For this review, take the finished solid that the model builds, in its own axes (mm). A direction names the side the tool comes from. Coordinates: 2 decimals unless noted, no trailing zeros. Loops run counter-clockwise (first coordinate to the right, second up) from the corner with the lowest first, then second, coordinate; pieces in that order, holes last.
1. To check wall thickness, follow probe 1 along X at (y, z) = (0.9, -50); probe 2 along X at (y, z) = (2.15, -27.5); probe 3 along X at (y, z) = (0.8, -27.5). State the ranges of each line that lie inside material, in increasing order.
2. Clearance check with flat-ended pins moving along their axes: P1, Ø1.6, axis at x = 35, z = -4, coming from the +Y side; P2, Ø1, axis at y = 0.5, z = -25, coming from the +X side; P3, Ø10, axis at x = 48.5, z = 5.5, coming from the +Y side; P4, Ø0.8, axis at y = 0.5, z = -22, coming from the -X side. State where each tip first meets the part, or that it passes through.
3. Take a section at B-B, the plane x = 9. State the section outline as (y, z) points, then the cut area to 3 significant figures.
4. Machinability: for faces 5 (the face through (70, 1, -31.9)), 6 (the face through (72, 0.125, -30)), 7 (the face through (-1, 1.2, -28)), which of the approach directions +Z, -Z, +X, -X, +Y, -Y give a long, thin tool a straight path to every point of the face, cutting with its end or side? Answer none if there is none.
5. Take a section at C-C, the plane y = 2.3. State the section outline as (x, z) points, then the cut area to 3 significant figures.
6. Take a section at A-A, the plane z = -27.5. State the section outline as (x, y) points (3 decimals).
7. Take a section at D-D, the plane x = 32.73. State the section outline as (y, z) points (3 decimals), then the cut area to 3 significant figures.
8. Mouldability with a two-part tool opening along Z and no side actions: class faces 1 (the face through (34, 1.5, -50)), 2 (the face through (76.15, 1.46, -27.4)), 3 (the face through (28.33, 1, 6)), 4 (the face through (70, 1, -23.1)) as pulls with the +Z half, pulls with the -Z half, needs draft (parallel to the pull), parting line crosses it, or undercut.
```python
from build123d import *

# Parameters (mm, degrees)
SKETCH1_W           = 68.5
SKETCH1_H           = 55
BOSS_EXTRUDE1_DEPTH = 1.5
SKETCH2_W           = 68.5
SKETCH2_H           = 55
SKETCH2_W_2         = 64.5
SKETCH2_H_2         = 51
BOSS_EXTRUDE2_DEPTH = 1.25
SKETCH3_R           = 1.25
SKETCH3_W           = 64.5
SKETCH3_H           = 40
CUT_EXTRUDE1_DEPTH  = 1.5
SKETCH4_W           = 23
SKETCH4_H           = 1.2
CUT_EXTRUDE2_DEPTH  = 3
SKETCH5_R           = 1.9
BOSS_EXTRUDE3_DEPTH = 2.625
SKETCH5_5_R         = 1.9
BOSS_EXTRUDE4_DEPTH = 1.55
BOSS_EXTRUDE5_DEPTH = 1.2


with BuildPart() as part:
    # Sketch1 → Boss-Extrude1 (new body)
    with BuildSketch(Plane(origin=(0, 0, 0), x_dir=(1, 0, 0), z_dir=(0, 1, 0))):
        with Locations((34.25, 27.5)):
            Rectangle(SKETCH1_W, SKETCH1_H)
    extrude(amount=BOSS_EXTRUDE1_DEPTH)

    # Sketch2 → Boss-Extrude2 (add)
    with BuildSketch(Plane(origin=(0, 1.5, 0), x_dir=(1, 0, 0), z_dir=(0, 1, 0))):
        with Locations((34.25, 27.5)):
            Rectangle(SKETCH2_W, SKETCH2_H)
        with Locations((34.25, 27.5)):
            Rectangle(SKETCH2_W_2, SKETCH2_H_2, mode=Mode.SUBTRACT)
    extrude(amount=BOSS_EXTRUDE2_DEPTH)

    # Sketch3 → Cut-Extrude1 (cut)
    with BuildSketch(Plane(origin=(0, 1.5, 0), x_dir=(1, 0, 0), z_dir=(0, 1, 0))):
        with Locations(Location((5, 50, 0), (0, 0, 270))):
            Circle(SKETCH3_R)
        with Locations(Location((63.5, 50, 0), (0, 0, 270))):
            Circle(SKETCH3_R)
        with Locations(Location((63.5, 5, 0), (0, 0, 270))):
            Circle(SKETCH3_R)
        with Locations(Location((5, 5, 0), (0, 0, 270))):
            Circle(SKETCH3_R)
        with Locations((34.25, 27.5)):
            Rectangle(SKETCH3_W, SKETCH3_H)
    extrude(amount=-CUT_EXTRUDE1_DEPTH, mode=Mode.SUBTRACT)

    # Sketch4 → Cut-Extrude2 (cut)
    with BuildSketch(Plane.ZY):
        with Locations((-27.5, 0.6)):
            Rectangle(SKETCH4_W, SKETCH4_H)
    extrude(amount=-CUT_EXTRUDE2_DEPTH, mode=Mode.SUBTRACT)

    # Sketch5 → Boss-Extrude3 (add)
    # profile 1 of 3: a face of its own
    with BuildSketch(Plane(origin=(0, 2.75, 0), x_dir=(1, 0, 0), z_dir=(0, 1, 0))):
        with BuildLine():
            Line((37.13, -11.52), (37.13, 0))
            Line((37.13, 0), (28.33, 0))
            Line((28.33, 0), (28.33, -11.52))
            ThreePointArc((28.33, -11.52), (32.73, -15.92), (37.13, -11.52))
        make_face()
        with Locations(Location((32.73, -11.52, 0), (0, 0, 270))):
            Circle(SKETCH5_R, mode=Mode.SUBTRACT)
    # profile 2 of 3: a face of its own
    with BuildSketch(Plane(origin=(0, 2.75, 0), x_dir=(1, 0, 0), z_dir=(0, 1, 0))):
        with BuildLine():
            Line((71.75, 31.9), (68.5, 31.9))
            Line((68.5, 31.9), (68.5, 23.1))
            Line((68.5, 23.1), (71.75, 23.1))
            ThreePointArc((71.75, 23.1), (76.15, 27.5), (71.75, 31.9))
        make_face()
        with Locations(Location((71.75, 27.5, 0), (0, 0, 270))):
            Circle(SKETCH5_R, mode=Mode.SUBTRACT)
    # profile 3 of 3: a face of its own
    with BuildSketch(Plane(origin=(0, 2.75, 0), x_dir=(1, 0, 0), z_dir=(0, 1, 0))):
        with BuildLine():
            Line((28.33, 55), (37.13, 55))
            Line((37.13, 55), (37.13, 66.52))
            ThreePointArc((37.13, 66.52), (32.73, 70.92), (28.33, 66.52))
            Line((28.33, 66.52), (28.33, 55))
        make_face()
        with Locations(Location((32.73, 66.52, 0), (0, 0, 270))):
            Circle(SKETCH5_R, mode=Mode.SUBTRACT)
    extrude(amount=-BOSS_EXTRUDE3_DEPTH)

    # Sketch5_5 → Boss-Extrude4 (add)
    with BuildSketch(Plane(origin=(0, 2.75, 0), x_dir=(1, 0, 0), z_dir=(0, 1, 0))):
        with BuildLine():
            Line((0, 23.1), (0, 31.9))
            Line((0, 31.9), (-6.29, 31.9))
            ThreePointArc((-6.29, 31.9), (-10.69, 27.5), (-6.29, 23.1))
            Line((-6.29, 23.1), (0, 23.1))
        make_face()
        with Locations(Location((-6.29, 27.5, 0), (0, 0, 270))):
            Circle(SKETCH5_5_R, mode=Mode.SUBTRACT)
    extrude(amount=-BOSS_EXTRUDE4_DEPTH)

    # Sketch6 → Boss-Extrude5 (add)
    with BuildSketch(Plane.XZ.offset(-1.2)):
        with BuildLine():
            Line((-6.29, -25.6), (-6.29, -23.1))
            ThreePointArc((-6.29, -23.1), (-10.69, -27.5), (-6.29, -31.9))
            Line((-6.29, -31.9), (-6.29, -29.4))
            ThreePointArc((-6.29, -29.4), (-8.19, -27.5), (-6.29, -25.6))
        make_face()
    extrude(amount=BOSS_EXTRUDE5_DEPTH)


solid = part.part
```
Results list:
1. probe 1: x = 0 to 3.75, 6.25 to 62.25, 64.75 to 68.5
1. probe 2: x = -10.69 to -8.19, -4.39 to 2, 66.5 to 69.85, 73.65 to 76.15
1. probe 3: x = -10.69 to -8.19, 66.5 to 69.85, 73.65 to 76.15
2. P1: stops at y = 1.5
2. P2: stops at x = 75.67
2. P3: passes through
2. P4: stops at x = 66.5
3. outline: (0, -55) - (2.75, -55) - (2.75, -53) - (1.5, -53) - (1.5, -47.5) - (0, -47.5) - close; (0, -7.5) - (1.5, -7.5) - (1.5, -2) - (2.75, -2) - (2.75, 0) - (0, 0) - close
3. area: 27.5 mm2
4. face 5: -Z, +X, +Y, -Y
4. face 6: +Z, -Z, +X, -Y
4. face 7: -Y
5. outline: (-6.29, -31.9) - (0, -31.9) - (0, -55) - (28.33, -55) - (28.33, -66.52) arc R4.4 ccw to (37.13, -66.52) - (37.13, -55) - (68.5, -55) - (68.5, -31.9) - (71.75, -31.9) arc R4.4 ccw to (71.75, -23.1) - (68.5, -23.1) - (68.5, 0) - (37.13, 0) - (37.13, 11.52) arc R4.4 ccw to (28.33, 11.52) - (28.33, 0) - (0, 0) - (0, -23.1) - (-6.29, -23.1) arc R4.4 ccw to start; hole circle Ø3.8 at (-6.29, -27.5); hole (2, -53) - (66.5, -53) - (66.5, -2) - (2, -2) - close; hole circle Ø3.8 at (32.73, -66.52); hole circle Ø3.8 at (32.73, 11.52); hole circle Ø3.8 at (71.75, -27.5)
5. area: 841 mm2
6. outline: (-10.69, 0) - (-8.19, 0) - (-8.19, 2.75) - (-10.69, 2.75) - close; (-4.39, 1.2) - (2, 1.2) - (2, 2.75) - (-4.39, 2.75) - close; (66.5, 0) - (68.5, 0) - (68.5, 0.125) - (69.85, 0.125) - (69.85, 2.75) - (66.5, 2.75) - close; (73.65, 0.125) - (76.15, 0.125) - (76.15, 2.75) - (73.65, 2.75) - close
7. outline: (0, -55) - (0.125, -55) - (0.125, -64.62) - (2.75, -64.62) - (2.75, -53) - (1.5, -53) - (1.5, -47.5) - (0, -47.5) - close; (0, -7.5) - (1.5, -7.5) - (1.5, -2) - (2.75, -2) - (2.75, 9.62) - (0.125, 9.62) - (0.125, 0) - (0, 0) - close; (0.125, -70.92) - (2.75, -70.92) - (2.75, -68.42) - (0.125, -68.42) - close; (0.125, 13.42) - (2.75, 13.42) - (2.75, 15.92) - (0.125, 15.92) - close
7. area: 91.1 mm2
8. face 1: undercut
8. face 2: parting line crosses it
8. face 3: needs draft
8. face 4: pulls with the +Z half
